Geometry check sheet. Reference: the model listing, model coordinates, mm. Coordinates: 2 decimals unless noted, no trailing zeros. Loops run counter-clockwise (first coordinate to the right, second up) from the corner with the lowest first, then second, coordinate; pieces in that order, holes last. Notation, with made-up numbers: (34, 23) -> (57, 23) arc R24 ccw to (57, 33) -> close; hole circle Ø11 at (67, 73.5). An arc over 180 degrees is marked (long way). Answer as a JSON object with one key per item and string values.
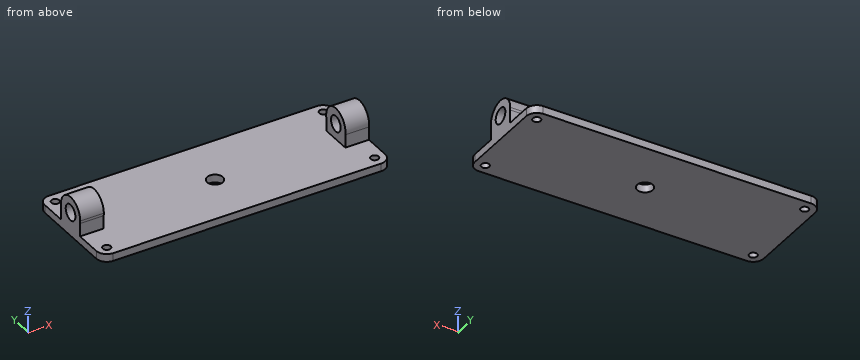
from build123d import *

# Parameters (mm, degrees)
F0_R     = 9.525
F1_DEPTH = 19.05
F3_DEPTH = 57.15
F5_DEPTH = 57.15


with BuildPart() as f1:
    # F0 (on Top) → F1 (new body)
    with BuildSketch(Plane.XY):
        with BuildLine():
            Line((349.25, 0), (19.05, 0))
            ThreePointArc((19.05, 0), (-13.4703841816, -13.4703841816), (0, 19.05))
            Line((0, 19.05), (0, 127))
            Line((0, 127), (-323.85, 127))
            ThreePointArc((-323.85, 127), (-341.8105122421, 119.5605122421), (-349.25, 101.6))
            Line((-349.25, 101.6), (-349.25, -101.6))
            ThreePointArc((-349.25, -101.6), (-341.8105122421, -119.5605122421), (-323.85, -127))
            Line((-323.85, -127), (323.85, -127))
            ThreePointArc((323.85, -127), (341.8105122421, -119.5605122421), (349.25, -101.6))
            Line((349.25, -101.6), (349.25, 0))
        make_face()
        with Locations((-323.85, -101.6)):
            Circle(F0_R, mode=Mode.SUBTRACT)
        with Locations((323.85, -101.6)):
            Circle(F0_R, mode=Mode.SUBTRACT)
        with Locations((-323.85, 101.6)):
            Circle(F0_R, mode=Mode.SUBTRACT)
        with BuildLine():
            ThreePointArc((0, 19.05), (13.4703841816, 13.4703841816), (19.05, 0))
            Line((19.05, 0), (349.25, 0))
            Line((349.25, 0), (349.25, 101.6))
            ThreePointArc((349.25, 101.6), (341.8105122421, 119.5605122421), (323.85, 127))
            Line((323.85, 127), (0, 127))
            Line((0, 127), (0, 19.05))
        make_face()
        with Locations((323.85, 101.6)):
            Circle(F0_R, mode=Mode.SUBTRACT)
    extrude(amount=-F1_DEPTH)

    # F2 (on face) → F3 (join)
    with BuildSketch(Plane(origin=(-349.25, 0, 0), x_dir=(0, -1, 0), z_dir=(-1, 0, 0))):
        with BuildLine():
            ThreePointArc((-37.5671066227, 31.75), (-24.5934442418, 9.0006443314), (1.73e-08, 0))
            ThreePointArc((1.73e-08, 0), (24.593444255, 9.0006443426), (37.5671066227, 31.75))
            ThreePointArc((37.5671066227, 31.75), (37.9665429182, 34.9138394833), (38.1, 38.1))
            ThreePointArc((38.1, 38.1), (-3.1861605167, 76.0665429182), (-37.5671066227, 31.75))
        make_face()
        with BuildLine():
            ThreePointArc((19.05, 38.1), (13.4703841816, 24.6296158184), (0, 19.05))
            ThreePointArc((0, 19.05), (-13.4703841816, 51.5703841816), (19.05, 38.1))
        make_face(mode=Mode.SUBTRACT)
        with BuildLine():
            Line((-37.5671066227, 0), (1.73e-08, 0))
            ThreePointArc((1.73e-08, 0), (-24.5934442418, 9.0006443314), (-37.5671066227, 31.75))
            Line((-37.5671066227, 31.75), (-37.5671066227, 0))
        make_face()
        with BuildLine():
            ThreePointArc((37.5671066227, 31.75), (24.593444255, 9.0006443426), (1.73e-08, 0))
            Line((1.73e-08, 0), (37.5671066227, 0))
            Line((37.5671066227, 0), (37.5671066227, 31.75))
        make_face()
    extrude(amount=-F3_DEPTH)

    # F4 (on face) → F5 (join)
    with BuildSketch(Plane.YZ.offset(349.25)):
        with BuildLine():
            ThreePointArc((37.5671066227, 31.75), (24.593444255, 9.0006443426), (1.73e-08, 0))
            Line((1.73e-08, 0), (37.5671066227, 0))
            Line((37.5671066227, 0), (37.5671066227, 31.75))
        make_face()
        with BuildLine():
            ThreePointArc((-37.5671066227, 31.75), (-24.5934442418, 9.0006443314), (1.73e-08, 0))
            ThreePointArc((1.73e-08, 0), (24.593444255, 9.0006443426), (37.5671066227, 31.75))
            ThreePointArc((37.5671066227, 31.75), (37.9665429182, 34.9138394833), (38.1, 38.1))
            ThreePointArc((38.1, 38.1), (-3.1861605167, 76.0665429182), (-37.5671066227, 31.75))
        make_face()
        with BuildLine():
            ThreePointArc((19.05, 38.1), (13.4703841816, 24.6296158184), (0, 19.05))
            ThreePointArc((0, 19.05), (-13.4703841816, 51.5703841816), (19.05, 38.1))
        make_face(mode=Mode.SUBTRACT)
        with BuildLine():
            Line((-37.5671066227, 0), (1.73e-08, 0))
            ThreePointArc((1.73e-08, 0), (-24.5934442418, 9.0006443314), (-37.5671066227, 31.75))
            Line((-37.5671066227, 31.75), (-37.5671066227, 0))
        make_face()
    extrude(amount=-F5_DEPTH)


solid = f1.part
1. Section check D-D, the plane x = -7. Record the boundary of the cut face in (y, z), then the cut area to 3 significant figures.
Evaluation:
{"outline": "(-127, -19.05) -> (-17.72, -19.05) -> (-17.72, 0) -> (-127, 0) -> close; (17.72, -19.05) -> (127, -19.05) -> (127, 0) -> (17.72, 0) -> close", "area": "4,160 mm^2"}
2. Depth check by flat-ended pin: P1, Ø16, axis at x = -329.5, z = 23, coming from the +Y side; P2, Ø2, axis at x = -60, y = 64.5, coming from the +Z side; P3, Ø16, axis at x = -319, z = 23.5, coming from the -Y side; P4, Ø3, axis at x = -279, z = 0.5, coming from the -Y side. Enter the tip coordinate at first touch or a pass-through.
Evaluation:
{"P1": "stops at y = 37.57", "P2": "stops at z = 0", "P3": "stops at y = -37.57", "P4": "stops at y = -127"}
3. Section check C-C, the plane z = 10. Record the boundary of the cut face in (x, y), then the cut area to 3 significant figures.
Evaluation:
{"outline": "(-349.25, -37.57) -> (-292.1, -37.57) -> (-292.1, 37.57) -> (-349.25, 37.57) -> close; (292.1, -37.57) -> (349.25, -37.57) -> (349.25, 37.57) -> (292.1, 37.57) -> close", "area": "8,590 mm^2"}
4. Section check A-A, the plane y = 0. Record the boundary of the cut face in (x, z), then the cut area to 3 significant figures.
Evaluation:
{"outline": "(-349.25, -19.05) -> (-19.05, -19.05) -> (-19.05, 0) -> (-292.1, 0) -> (-292.1, 19.05) -> (-349.25, 19.05) -> close; (-349.25, 57.15) -> (-292.1, 57.15) -> (-292.1, 76.2) -> (-349.25, 76.2) -> close; (19.05, -19.05) -> (349.25, -19.05) -> (349.25, 19.05) -> (292.1, 19.05) -> (292.1, 0) -> (19.05, 0) -> close; (292.1, 57.15) -> (349.25, 57.15) -> (349.25, 76.2) -> (292.1, 76.2) -> close", "area": "16,900 mm^2"}
5. Section check B-B, the plane x = -302.5. Record the boundary of the cut face in (y, z), then the cut area to 3 significant figures.
Evaluation:
{"outline": "(-127, -19.05) -> (127, -19.05) -> (127, 0) -> (37.57, 0) -> (37.57, 31.75) arc R38.1 ccw (long way) to (-37.57, 31.75) -> (-37.57, 0) -> (-127, 0) -> close; hole circle Ø38.1 at (0, 38.1)", "area": "8,850 mm^2"}
6. Thickness scan on probe 1 along X at (y, z) = (101, -14); probe 2 along Y at (x, z) = (323, -8); probe 3 along Z at (x, y) = (-329, 0). Record the ranges inside material, lowest first. Write a range as from..to.
Evaluation:
{"probe 1": "x = -349.25..-333.36, -314.34..314.34, 333.36..349.25", "probe 2": "y = -127..-111.09, -92.11..92.11, 111.09..127", "probe 3": "z = -19.05..19.05, 57.15..76.2"}
